from build123d import *

# Parameters (mm, degrees)
CYLINDER963_R          = 2.5
CYLINDER963_DEPTH      = 20
CYLINDER961_R          = 2.5
CYLINDER961_DEPTH      = 20
CYLINDER962_R          = 74
CYLINDER962_DEPTH      = 10
BOX477_W               = 51
BOX477_H               = 24
BOX477_DEPTH           = 6
CUT444_PLACEMENT_ANGLE = 90


with BuildPart() as obj1:
    # Cylinder963 → Cylinder963 (new body)
    with BuildSketch(Plane(origin=(-86, -10, 66), x_dir=(1, 0, 0), z_dir=(0, 0, 1))):
        Circle(CYLINDER963_R)
    extrude(amount=CYLINDER963_DEPTH)


with BuildPart() as compound519:
    # Cylinder961 → Cylinder961 (new body)
    with BuildSketch(Plane(origin=(-102, -10, 66), x_dir=(1, 0, 0), z_dir=(0, 0, 1))):
        Circle(CYLINDER961_R)
    extrude(amount=CYLINDER961_DEPTH)

    # Compound519: union obj1
    add(obj1.part)


with BuildPart() as obj2:
    # Cylinder962 → Cylinder962 (new body)
    with BuildSketch(Plane.XY.offset(72)):
        Circle(CYLINDER962_R)
    extrude(amount=CYLINDER962_DEPTH)


with BuildPart() as cut444:
    # Box477 → Box477 (new body)
    with BuildSketch(Plane(origin=(-112, -24, 76), x_dir=(1, 0, 0), z_dir=(0, 0, 1))):
        with Locations((25.5, 12)):
            Rectangle(BOX477_W, BOX477_H)
    extrude(amount=BOX477_DEPTH)

    # Cut445: cut obj2
    add(obj2.part, mode=Mode.SUBTRACT)

    # Cut444: cut Compound519
    add(compound519.part, mode=Mode.SUBTRACT)


with BuildPart() as cut444_1:
    # Cut444 placement: moved
    add(cut444.part.rotate(Axis((0, 0, 0), (0, 0, 1)), CUT444_PLACEMENT_ANGLE))


solid = cut444_1.part
For this review, take the finished solid that the model builds, in its own axes (mm). Round coordinates to 2 decimals unless told otherwise and drop trailing zeros. Loops run counter-clockwise (first coordinate to the right, second up) from the corner with the lowest first, then second, coordinate; pieces in that order, holes last. Notation, with made-up numbers: (71, -3) - (94, -3) arc R22 ccw to (94, 15) - close; hole circle Ø11 at (22.5, 72). An arc over 180 degrees is marked (long way). Answer as CSV lines item,"result".
(1) Consider section A-A on y = -102. Give the boundary of the cut face in (x, z).
Checked values:
outline,"(0, 76) - (7.5, 76) - (7.5, 82) - (0, 82) - close; (12.5, 76) - (24, 76) - (24, 82) - (12.5, 82) - close"
(2) Consider section D-D on x = 21. Give the boundary of the cut face in (y, z), then the cut area to 3 significant figures.
Checked values:
outline,"(-112, 76) - (-70.96, 76) - (-70.96, 82) - (-112, 82) - close"
area,"246 mm2"
(3) Mouldability with a two-part tool opening along X and no side actions: class faces 1 (the face through (12, -112, 79)), 2 (the face through (12.22, -100.85, 78.96)), 3 (the face through (24, -91, 79)), 4 (the face through (0, -93, 79)) as +X half, -X half, draft (parallel to the pull), parting line (faces both ways), or undercut.
Checked values:
face 1,"draft"
face 2,"undercut"
face 3,"+X half"
face 4,"-X half"
(4) Insertion check: P1, Ø1.5, axis at x = 4, z = 77.5, coming from the +Y side; P2, Ø2, axis at x = 20, z = 78, coming from the +Y side. Each pin has a flat end and moves straight along its axis. Give the tip position at first contact, or say it passes through.
Checked values:
P1,"stops at y = -73.85"
P2,"stops at y = -70.96"
(5) Wall thickness on line 1 (X direction, y = -86, z = 78.7); line 2 (Y direction, x = 10, z = 77.8); line 3 (Y direction, x = 12, z = 79.6): over which ranges is each line inside the solid? List them lowest first.
Checked values:
line 1,"x = 0 to 7.5, 12.5 to 24"
line 2,"y = -112 to -104.5, -99.5 to -88.5, -83.5 to -73.32"
line 3,"y = -112 to -103.5, -100.5 to -87.5, -84.5 to -73.02"
(6) Consider section B-B on x = 10. Give the boundary of the cut face in (y, z).
Checked values:
outline,"(-112, 76) - (-104.5, 76) - (-104.5, 82) - (-112, 82) - close; (-99.5, 76) - (-88.5, 76) - (-88.5, 82) - (-99.5, 82) - close; (-83.5, 76) - (-73.32, 76) - (-73.32, 82) - (-83.5, 82) - close"
(7) Consider section C-C on z = 78.2. Give the boundary of the cut face in (x, y).
Checked values:
outline,"(0, -112) - (24, -112) - (24, -70) arc R74 cw to (0, -74) - close; hole circle Ø5 at (10, -102); hole circle Ø5 at (10, -86)"
